Autodesk Inventor part; units mm, degrees
ref_plane "YZ Plane" through (0, 0, 0) normal (1, 0, 0) x (0, 1, 0)
ref_plane "XZ Plane" through (0, 0, 0) normal (0, 1, 0) x (-1, 0, 0)
ref_plane "XY Plane" through (0, 0, 0) normal (0, 0, 1) x (1, 0, 0)
sketch "草圖1" plane through (0, 0, 0) normal (0, 0, 1) x (1, 0, 0)
  line L0 (-1.7305, 1.0027) -> (-17.0365, 9.8719)
  line L1 (-18.7669, 10.8747) -> (-38.873, 1.2756)
  line L2 (-40.6779, 0.4139) -> (-1.9999, 0.0203)
  line L3 (8.4583, -2.0862) -> (-44.617, -1.5461)
  line L4 (-19.6286, 12.6795) -> (-43.3233, 1.3672)
  line L5 (7.8765, -2.2526) -> (-17.7642, 12.6051)
  arc A0 (-17.7642, 12.6051) -> (-19.6286, 12.6795) centre (-18.7669, 10.8747) ccw
  arc A1 (-20.5718, 10.013) -> (-17.0365, 9.8719) centre (-18.7669, 10.8747) ccw
  arc A2 (-1.7305, 1.0027) -> (-1.9999, 0.0203) centre (0, 0) ccw
  arc A3 (-0.0203, -1.9999) -> (1.0027, 1.7305) centre (0, 0) ccw
  arc A4 (-41.5396, 2.2188) -> (-40.6982, -1.586) centre (-40.6779, 0.4139) ccw
  arc A5 (-38.678, 0.3936) -> (-38.873, 1.2756) centre (-40.6779, 0.4139) ccw
  dimension "d0" = 21.69
  dimension "d1" = 24.28
  dimension "d2" = 40.68
extrude "擠出1" add sketch "草圖1" along normal blind 1 contours L3 A4 L4 A0 L5 A3
sketch "草圖2" plane through (0, 0, 1) normal (0, 0, 1) x (1, 0, 0)
  arc A0 (-20.5718, 10.013) -> (-17.0365, 9.8719) centre (-18.7669, 10.8747) ccw
  circle A1 centre (-18.7669, 10.8747) radius 1
  circle A2 centre (0, 0) radius 1
  arc A3 (-38.678, 0.3936) -> (-38.873, 1.2756) centre (-40.6779, 0.4139) ccw
  circle A4 centre (-40.6779, 0.4139) radius 1
  dimension "d8" = 2
  dimension "d9" = 2
  dimension "d10" = 2
extrude "擠出2" cut sketch "草圖2" against normal blind 10
properties part number "三角塊2"
Geometry: final body of the model. Coordinates: model frame, mm. A direction names the side the tool comes from. Round coordinates to 2 decimals unless told otherwise and drop trailing zeros. Write each loop counter-clockwise with the first axis right and the second up, starting at its lowest first coordinate (ties: lowest second). Pieces come first, ordered by that corner, then holes. Notation, with made-up numbers: M 13,0.5 L 17,0.5 A14 ccw 17,8.5 Z; hole C -9,-3.75 d11. An arc over 180 degrees is marked long. Write item = value, one per line.
Item 1: Pin query (flat end, axial travel): P1, Ø2.5, axis at x = -18.77, y = 10.87, coming from the -Z side; P2, Ø2, axis at x = -24.5, y = 3, coming from the -Z side. Return the tip coordinate at first contact, or that it passes through.
Findings:
P1 = 0
P2 = through
Item 2: Pull-direction query (X, two-part tool) for faces 1 (the face through (-1.93, 0.52, 0.49)), 2 (the face through (-30.431, 7.522, 0.493)), 3 (the face through (-20, -1, 0)); classes: pulls with the +X half, pulls with the -X half, needs draft (parallel to the pull), parting line crosses it, or undercut.
Findings:
face_1 = undercut
face_2 = pulls with the -X half
face_3 = needs draft
Item 3: Section query A-A on x = -33.5. Return loops of the section in (y, z), then the cut area to 3 significant figures.
Findings:
outline = M -1.66,0 L 0.34,0 L 0.34,1 L -1.66,1 Z; M 3.84,0 L 6.06,0 L 6.06,1 L 3.84,1 Z
area = 4.22 mm^2
Item 4: Material intervals for line 1 along X through (y, z) = (0.5, 0.4); line 2 along X through (y, z) = (9.5, 0.1); line 3 along X through (y, z) = (6.75, 0.5), sorted ascending. Write a range as [from, to].
Findings:
line_1 = [-42.68, -41.67], [-39.68, -38.68], [-1.94, -0.87], [0.87, 1.94]
line_2 = [-26.29, -21.65], [-20.22, -17.31], [-16.39, -12.41]
line_3 = [-32.05, -27.41], [-11.65, -7.66]
Item 5: Access query for faces 4 (the face through (-38.726, 0.852, 0.493)), 5 (the face through (-20, -1, 1)). Directions: +Z, -Z, +X, -X, +Y, -Y. A direction counts if a zero-diameter tool reaches every point of the face in a straight line with its end or side. Return the directions, or none.
Findings:
face_4 = +Z, -Z
face_5 = +Z, +X, -X, +Y, -Y
Item 6: Section query C-C on z = 0.6. Return loops of the section in (x, y).
Findings:
outline = M -41.54,2.22 A2 ccw -40.7,-1.59 L -0.02,-2 A2 ccw 1,1.73 L -17.76,12.61 A2 ccw -19.63,12.68 Z; hole C -40.68,0.41 d2; hole M -38.87,1.28 A2 cw -38.68,0.39 L -2,0.02 A2 cw -1.73,1 L -17.04,9.87 A2 cw -20.57,10.01 Z; hole C -18.77,10.87 d2; hole C 0,0 d2
Item 7: Section query B-B on y = 6.5. Return loops of the section in (x, z).
Findings:
outline = M -32.57,0 L -27.93,0 L -27.93,1 L -32.57,1 Z; M -11.22,0 L -7.23,0 L -7.23,1 L -11.22,1 Z
